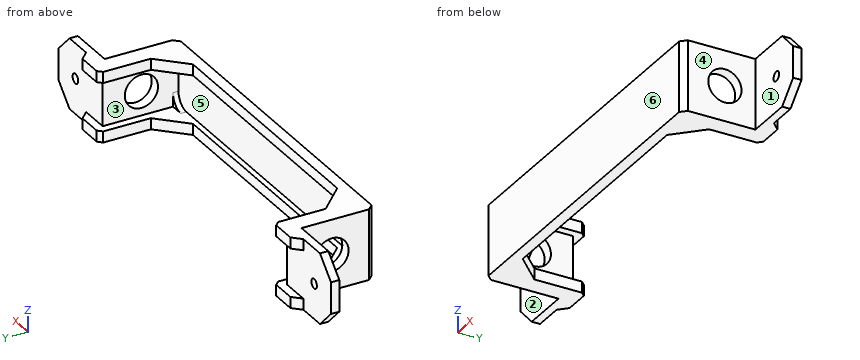
```python
from build123d import *

# Parameters (mm, degrees)
SKETCH1_W           = 125
SKETCH1_H           = 25.4
BOSS_EXTRUDE1_DEPTH = 4
SKETCH2_W           = 117
SKETCH2_H           = 17.4
CUT_EXTRUDE1_DEPTH  = 2
FILLET1_R           = 5
SKETCH3_W           = 4
SKETCH3_H           = 25.4
BOSS_EXTRUDE2_DEPTH = 25.4
CHAMFER1_SIZE       = 2
SKETCH4_R           = 6
CUT_EXTRUDE3_DEPTH  = 135.4
SKETCH5_W           = 25.4
SKETCH5_H           = 3
BOSS_EXTRUDE3_DEPTH = 24
SKETCH6_W           = 25.4
SKETCH6_H           = 3
BOSS_EXTRUDE4_DEPTH = 24
BOSS_EXTRUDE5_DEPTH = 4
BOSS_EXTRUDE6_DEPTH = 4
SKETCH9_R           = 1.75
CUT_EXTRUDE4_DEPTH  = 4
CHAMFER2_SIZE       = 7
BOSS_EXTRUDE7_DEPTH = 4
BOSS_EXTRUDE8_DEPTH = 4
CHAMFER3_SIZE       = 1.5


with BuildPart() as part:
    # Sketch1 → Boss-Extrude1 (new body)
    with BuildSketch(Plane(origin=(0, 0, 0), x_dir=(1, 0, 0), z_dir=(0, 1, 0))):
        Rectangle(SKETCH1_W, SKETCH1_H)
    extrude(amount=BOSS_EXTRUDE1_DEPTH)

    # Sketch2 → Cut-Extrude1 (cut)
    with BuildSketch(Plane(origin=(0, 4, 0), x_dir=(1, 0, 0), z_dir=(0, 1, 0))):
        Rectangle(SKETCH2_W, SKETCH2_H)
    extrude(amount=-CUT_EXTRUDE1_DEPTH, mode=Mode.SUBTRACT)

    # Fillet1
    fillet1_edges = [part.edges().sort_by_distance(p)[0] for p in [
        (58.5, 3, -8.7),
        (58.5, 3, 8.7),
        (-58.5, 3, 8.7),
        (-58.5, 3, -8.7),
    ]]
    fillet(fillet1_edges, radius=FILLET1_R)

    # Sketch3 → Boss-Extrude2 (add)
    with BuildSketch(Plane(origin=(0, 4, 0), x_dir=(1, 0, 0), z_dir=(0, 1, 0))):
        with Locations((60.5, 0)):
            Rectangle(SKETCH3_W, SKETCH3_H)
        with Locations((-60.5, 0)):
            Rectangle(SKETCH3_W, SKETCH3_H)
    extrude(amount=BOSS_EXTRUDE2_DEPTH)

    # Chamfer1
    chamfer1_edges = [part.edges().sort_by_distance(p)[0] for p in [
        (-62.5, 0, 0),
        (62.5, 0, 0),
    ]]
    chamfer(chamfer1_edges, length=CHAMFER1_SIZE)

    # Sketch4 → Cut-Extrude3 (cut)
    with BuildSketch(Plane(origin=(62.5, 0, 0), x_dir=(0, 0, -1), z_dir=(1, 0, 0))):
        with Locations((0, 15.4)):
            Circle(SKETCH4_R)
    extrude(amount=-CUT_EXTRUDE3_DEPTH, mode=Mode.SUBTRACT)

    # Sketch5 → Boss-Extrude3 (add)
    with BuildSketch(Plane.ZY.offset(62.5)):
        with Locations((0, 27.9)):
            Rectangle(SKETCH5_W, SKETCH5_H)
    extrude(amount=BOSS_EXTRUDE3_DEPTH)

    # Sketch6 → Boss-Extrude4 (add)
    with BuildSketch(Plane(origin=(62.5, 0, 0), x_dir=(0, 0, -1), z_dir=(1, 0, 0))):
        with Locations((0, 27.9)):
            Rectangle(SKETCH6_W, SKETCH6_H)
    extrude(amount=BOSS_EXTRUDE4_DEPTH)

    # Sketch7 → Boss-Extrude5 (add)
    with BuildSketch(Plane.XY.offset(12.7)):
        Polygon((-58.5, 16.7), (-45.8, 4), (-58.5, 4), align=None)
        Polygon((58.5, 16.7), (45.8, 4), (58.5, 4), align=None)
    extrude(amount=-BOSS_EXTRUDE5_DEPTH)

    # Sketch8 → Boss-Extrude6 (add)
    with BuildSketch(Plane(origin=(0, 0, -12.7), x_dir=(-1, 0, 0), z_dir=(0, 0, -1))):
        Polygon((-58.5, 16.7), (-45.8, 4), (-58.5, 4), align=None)
        Polygon((58.5, 16.7), (45.8, 4), (58.5, 4), align=None)
    extrude(amount=-BOSS_EXTRUDE6_DEPTH)

    # Sketch9 → Cut-Extrude4 (cut)
    with BuildSketch(Plane(origin=(0, 29.4, 0), x_dir=(1, 0, 0), z_dir=(0, 1, 0))):
        with Locations(Location((75.8, 0, 0), (0, 0, 270))):
            Circle(SKETCH9_R)
        with Locations(Location((-75.8, 0, 0), (0, 0, 270))):
            Circle(SKETCH9_R)
    extrude(amount=-CUT_EXTRUDE4_DEPTH, mode=Mode.SUBTRACT)

    # Chamfer2
    chamfer2_edges = [part.edges().sort_by_distance(p)[0] for p in [
        (-86.5, 27.9, -12.7),
        (-86.5, 27.9, 12.7),
        (86.5, 27.9, 12.7),
        (86.5, 27.9, -12.7),
    ]]
    chamfer(chamfer2_edges, length=CHAMFER2_SIZE)

    # Sketch10 → Boss-Extrude7 (add)
    with BuildSketch(Plane(origin=(0, 0, -12.7), x_dir=(-1, 0, 0), z_dir=(0, 0, -1))):
        Polygon((-69, 29.4), (-66, 32.4), (-55.5, 32.4), (-55.5, 13.7), (-58.5, 16.7), (-58.5, 29.4), align=None)
        Polygon((69, 29.4), (66, 32.4), (55.5, 32.4), (55.5, 13.7), (58.5, 16.7), (58.5, 29.4), align=None)
    extrude(amount=-BOSS_EXTRUDE7_DEPTH)

    # Sketch11 → Boss-Extrude8 (add)
    with BuildSketch(Plane.XY.offset(12.7)):
        Polygon((69, 29.4), (66, 32.4), (55.5, 32.4), (55.5, 13.7), (58.5, 16.7), (58.5, 29.4), align=None)
        Polygon((-69, 29.4), (-66, 32.4), (-55.5, 32.4), (-55.5, 13.7), (-58.5, 16.7), (-58.5, 29.4), align=None)
    extrude(amount=-BOSS_EXTRUDE8_DEPTH)

    # Chamfer3
    chamfer3_edges = [part.edges().sort_by_distance(p)[0] for p in [
        (55.5, 32.4, -10.7),
        (-55.5, 32.4, -10.7),
        (55.5, 32.4, 10.7),
        (-55.5, 32.4, 10.7),
    ]]
    chamfer(chamfer3_edges, length=CHAMFER3_SIZE)


solid = part.part
```
Input: part model. Units: mm. Frame: model coordinates. Face numbers are marked on the shaded views. A direction names the side the tool comes from. Give positions to 0.01 mm unless a question says otherwise; leave off trailing zeros. Write each loop counter-clockwise with the first axis right and the second up, starting at its lowest first coordinate (ties: lowest second). Pieces come first, ordered by that corner, then holes. Notation, with made-up numbers: (72, -23.75) - (107, -23.75) arc R15 ccw to (107, -11.75) - close; hole circle Ø6 at (46.5, 87). An arc over 180 degrees is marked (long way). Write item = value, one per line. Start each with the question number.
1) Reachability of the marked faces 1, 2 and 3 from +Z, -Z, +X, -X, +Y, -Y: full face, straight path, thin tool, end or side. Return the list, or none.
2) Pin query (flat end, axial travel): pin 1 (3 mm diameter, centred on x = -75.8, z = 0, fed in from -Y); pin 2 (7.5 mm diameter, centred on y = 18, z = 0.5, fed in from -X); pin 3 (12 mm diameter, centred on y = 6, z = -7.5, fed in from +X); pin 4 (4.5 mm diameter, centred on y = 26.5, z = 10, fed in from +X). Return the tip coordinate at first contact, or that it passes through.
3) Cut plane C-C (y = 12). Return loops of the section in (x, z).
4) Draft query along X for the marked faces 4, 5 and 6. Return one class per face: pulls with the +X half, pulls with the -X half, needs draft (parallel to the pull), parting line crosses it, or undercut.
5) Cut plane D-D (z = -10.75). Return loops of the section in (x, y), and give its area (3 significant figures).
6) Cut plane A-A (x = 75.8). Return loops of the section in (y, z), and give its area (3 significant figures).
7) Material intervals for L1, parallel to X at y = 27.35, z = 0; L2, parallel to X at y = 22.5, z = -6; L3, parallel to X at y = 26.5, z = 5, sorted ascending. Write a range as [from, to].
8) Cut plane B-B (z = 0). Give the number of separate pieces and of enclosed holes in the cut face, and give its area (3 significant figures).
Answers follow:
q1.face_1 = +Z, -Z, +X, -Y
q1.face_2 = +Z, -Z, -X, -Y
q1.face_3 = +Y
q2.pin_1 = through
q2.pin_2 = -62.5
q2.pin_3 = 62.5
q2.pin_4 = 84.45
q3.outline = (-62.5, -12.7) - (-53.8, -12.7) - (-53.8, -8.7) - (-58.5, -8.7) - (-58.5, -4.94) - (-62.5, -4.94) - close; (-62.5, 4.94) - (-58.5, 4.94) - (-58.5, 8.7) - (-53.8, 8.7) - (-53.8, 12.7) - (-62.5, 12.7) - close; (53.8, -12.7) - (62.5, -12.7) - (62.5, -4.94) - (58.5, -4.94) - (58.5, -8.7) - (53.8, -8.7) - close; (53.8, 8.7) - (58.5, 8.7) - (58.5, 4.94) - (62.5, 4.94) - (62.5, 12.7) - (53.8, 12.7) - close
q4.face_4 = pulls with the +X half
q4.face_5 = undercut
q4.face_6 = needs draft
q5.outline = (-81.45, 26.4) - (-62.5, 26.4) - (-62.5, 2) - (-60.5, 0) - (60.5, 0) - (62.5, 2) - (62.5, 26.4) - (81.45, 26.4) - (81.45, 29.4) - (69, 29.4) - (66, 32.4) - (57, 32.4) - (55.5, 30.9) - (55.5, 13.7) - (45.8, 4) - (-45.8, 4) - (-55.5, 13.7) - (-55.5, 30.9) - (-57, 32.4) - (-66, 32.4) - (-69, 29.4) - (-81.45, 29.4) - close
q5.area = 1,130 mm^2
q6.outline = (26.4, -12.7) - (29.4, -12.7) - (29.4, -1.75) - (26.4, -1.75) - close; (26.4, 1.75) - (29.4, 1.75) - (29.4, 12.7) - (26.4, 12.7) - close
q6.area = 65.7 mm^2
q7.L1 = [-86.5, -77.55], [-74.05, -58.5], [58.5, 74.05], [77.55, 86.5]
q7.L2 = [-62.5, -58.5], [58.5, 62.5]
q7.L3 = [-86.5, -58.5], [58.5, 86.5]
q8.separate_pieces = 5
q8.enclosed_holes = 0
q8.area = 492 mm^2
